For this review, take the finished solid that the model builds, in its own axes (mm). A direction names the side the tool comes from. Give positions to 0.01 mm unless a question says otherwise; leave off trailing zeros. Loops run counter-clockwise (first coordinate to the right, second up) from the corner with the lowest first, then second, coordinate; pieces in that order, holes last. Notation, with made-up numbers: (83, -0.5) -> (105, -0.5) arc R27 cw to (105, 20.5) -> close; hole circle Ø9 at (67, 40). An arc over 180 degrees is marked (long way). Write each question's results on one line, items separated by ' | '. Start each with the question number.
```python
from build123d import *

# Parameters (mm, degrees)
SKETCH1_W               = 56
SKETCH1_H               = 7.25
SKETCH1_R               = 1.6
SKETCH1_W_2             = 5
SKETCH1_H_2             = 16.75
SKETCH1_W_3             = 11.5
BOSS_EXTRUDE1_DEPTH     = 3
SKETCH2_W               = 8
SKETCH2_H               = 7
BOSS_EXTRUDE2_DEPTH     = 3
FILLET1_R               = 2
SKETCH3_W               = 16
SKETCH3_H               = 16
BOSS_EXTRUDE3_DEPTH     = 4
BOSS_EXTRUDE4_DEPTH     = 3
BOSS_EXTRUDE5_DEPTH     = 2
BOSS_EXTRUDE6_DEPTH     = 2
CHAMFER1_SIZE           = 3
SKETCH8_W               = 8
SKETCH8_H               = 10
CUT_EXTRUDE1_DEPTH      = 10
SKETCH9_R               = 1.45
BOSS_EXTRUDE7_DEPTH     = 3
SKETCH11_R              = 2.5
BOSS_EXTRUDE8_DEPTH     = 1.5
CUT_EXTRUDE3_DEPTH      = 74.518705103
CUT_EXTRUDE3_DEPTH_BACK = 2
CUT_EXTRUDE4_DEPTH      = 72.979163652
CUT_EXTRUDE4_DEPTH_BACK = 2


with BuildPart() as part:
    # Sketch1 → Boss-Extrude1 (new body)
    # profile 1 of 4: a face of its own
    with BuildSketch(Plane(origin=(0, 0, 0), x_dir=(1, 0, 0), z_dir=(0, 1, 0))):
        with Locations((-28, 3.625)):
            Rectangle(SKETCH1_W, SKETCH1_H)
        with Locations(Location((-7.6, 3.625, 0), (0, 0, 270))):
            Circle(SKETCH1_R, mode=Mode.SUBTRACT)
        with Locations(Location((-48.4, 3.625, 0), (0, 0, 270))):
            Circle(SKETCH1_R, mode=Mode.SUBTRACT)
    # profile 2 of 4: a face of its own
    with BuildSketch(Plane(origin=(0, 0, 0), x_dir=(1, 0, 0), z_dir=(0, 1, 0))):
        with Locations((-2.5, -8.375)):
            Rectangle(SKETCH1_W_2, SKETCH1_H_2)
    # profile 3 of 4: a face of its own
    with BuildSketch(Plane(origin=(0, 0, 0), x_dir=(1, 0, 0), z_dir=(0, 1, 0))):
        with Locations((5.75, -8.375)):
            Rectangle(SKETCH1_W_3, SKETCH1_H_2)
    # profile 4 of 4: a face of its own
    with BuildSketch(Plane(origin=(0, 0, 0), x_dir=(1, 0, 0), z_dir=(0, 1, 0))):
        with Locations((-10.75, -8.375)):
            Rectangle(SKETCH1_W_3, SKETCH1_H_2)
    extrude(amount=BOSS_EXTRUDE1_DEPTH)

    # Sketch2 → Boss-Extrude2 (add)
    # profile 1 of 2: a face of its own
    with BuildSketch(Plane(origin=(0, 3, 0), x_dir=(1, 0, 0), z_dir=(0, 1, 0))):
        with Locations((-48.4, 3.625)):
            Rectangle(SKETCH2_W, SKETCH2_H)
        Polygon((-46.725684219, 0.725), (-45.051368439, 3.625), (-46.725684219, 6.525), (-50.074315781, 6.525), (-51.748631561, 3.625), (-50.074315781, 0.725), align=None, mode=Mode.SUBTRACT)
    # profile 2 of 2: a face of its own
    with BuildSketch(Plane(origin=(0, 3, 0), x_dir=(1, 0, 0), z_dir=(0, 1, 0))):
        with Locations((-7.6, 3.625)):
            Rectangle(SKETCH2_W, SKETCH2_H)
        Polygon((-5.925684219, 0.725), (-4.251368439, 3.625), (-5.925684219, 6.525), (-9.274315781, 6.525), (-10.948631561, 3.625), (-9.274315781, 0.725), align=None, mode=Mode.SUBTRACT)
    extrude(amount=BOSS_EXTRUDE2_DEPTH)

    # Fillet1
    fillet1_edges = [part.edges().sort_by_distance(p)[0] for p in [
        (-44.4, 4.5, -0.125),
        (-44.4, 4.5, -7.125),
        (-52.4, 4.5, -7.125),
        (-52.4, 4.5, -0.125),
        (-3.6, 4.5, -0.125),
        (-3.6, 4.5, -7.125),
        (-11.6, 4.5, -7.125),
        (-11.6, 4.5, -0.125),
    ]]
    fillet(fillet1_edges, radius=FILLET1_R)

    # Sketch3 → Boss-Extrude3 (add)
    with BuildSketch(Plane(origin=(0, 3, 0), x_dir=(1, 0, 0), z_dir=(0, 1, 0))):
        with Locations((3.5, -8.75)):
            Rectangle(SKETCH3_W, SKETCH3_H)
    extrude(amount=BOSS_EXTRUDE3_DEPTH)

    # Sketch5 → Boss-Extrude4 (add)
    with BuildSketch(Plane.ZY.offset(4.5)):
        Polygon((-9.25, 7), (0.75, 7), (16.75, 7), (30.75, 7), (30.75, 37), (-9.25, 37), align=None)
    extrude(amount=-BOSS_EXTRUDE4_DEPTH)

    # Sketch6 → Boss-Extrude5 (add)
    with BuildSketch(Plane.XY.offset(16.75)):
        Polygon((-1.5, 37), (0, 37), (11.5, 7), (-1.5, 7), align=None)
    extrude(amount=-BOSS_EXTRUDE5_DEPTH)

    # Sketch7 → Boss-Extrude6 (add)
    with BuildSketch(Plane(origin=(0, 0, 0.75), x_dir=(-1, 0, 0), z_dir=(0, 0, -1))):
        Polygon((1.5, 37), (0, 37), (-11.5, 7), (1.5, 7), align=None)
    extrude(amount=-BOSS_EXTRUDE6_DEPTH)

    # Chamfer1
    chamfer1_edges = [part.edges().sort_by_distance(p)[0] for p in [
        (-3, 7, -9.25),
        (-3, 37, -9.25),
        (-3, 37, 30.75),
        (-3, 7, 30.75),
    ]]
    chamfer(chamfer1_edges, length=CHAMFER1_SIZE)

    # Sketch8 → Cut-Extrude1 (cut)
    with BuildSketch(Plane(origin=(-1.5, 0, 0), x_dir=(0, 0, -1), z_dir=(1, 0, 0))):
        with Locations((-8.75, 22)):
            Rectangle(SKETCH8_W, SKETCH8_H)
    extrude(amount=-CUT_EXTRUDE1_DEPTH, mode=Mode.SUBTRACT)

    # Sketch9 → Boss-Extrude7 (add)
    with BuildSketch(Plane(origin=(-1.5, 0, 0), x_dir=(0, 0, -1), z_dir=(1, 0, 0))):
        with Locations(Location((-8.75, 31.75, 0), (0, 0, 180))):
            Circle(SKETCH9_R)
        with Locations(Location((-8.75, 12.25, 0), (0, 0, 180))):
            Circle(SKETCH9_R)
    extrude(amount=BOSS_EXTRUDE7_DEPTH)

    # Sketch11 → Boss-Extrude8 (add)
    with BuildSketch(Plane(origin=(-1.5, 0, 0), x_dir=(0, 0, -1), z_dir=(1, 0, 0))):
        with Locations(Location((-8.75, 31.75, 0), (0, 0, 180))):
            Circle(SKETCH11_R)
        with Locations(Location((-8.75, 12.25, 0), (0, 0, 180))):
            Circle(SKETCH11_R)
    extrude(amount=BOSS_EXTRUDE8_DEPTH)

    # Sketch13 → Cut-Extrude3 (cut, two sides: drawn at the far end of the back side and taken through both)
    with BuildSketch(Plane(origin=(0, 0, 0.75), x_dir=(-1, 0, 0), z_dir=(0, 0, -1)).offset(-CUT_EXTRUDE3_DEPTH_BACK)):
        Polygon((0, 185.220530074), (0, 37), (0, 13.52173913), (-9, 13.52173913), (-157.220530074, 13.52173913), (-375.851096448, 213.716588185), (-218.630566375, 385.415379128), align=None)
    extrude(amount=CUT_EXTRUDE3_DEPTH + CUT_EXTRUDE3_DEPTH_BACK, mode=Mode.SUBTRACT)

    # Sketch14 → Cut-Extrude4 (cut, two sides: drawn at the far end of the back side and taken through both)
    with BuildSketch(Plane.XY.offset(16.75).offset(-CUT_EXTRUDE4_DEPTH_BACK)):
        Polygon((0, 185.220530074), (0, 37), (0, 13.52173913), (9, 13.52173913), (157.220530074, 13.52173913), (375.851096448, 213.716588185), (218.630566375, 385.415379128), align=None)
    extrude(amount=CUT_EXTRUDE4_DEPTH + CUT_EXTRUDE4_DEPTH_BACK, mode=Mode.SUBTRACT)


solid = part.part
```
1. We need section C-C (x = -7.6). Write out the cut boundary in (y, z) (3 decimals).
2. For pin 1 Ø8 at (y, z) = (25.5, 20) entering from -X; pin 2 Ø4 at (x, y) = (3.5, 24) entering from -Z; pin 3 Ø8 at (x, y) = (4, 12) entering from -Z; pin 4 Ø1.5 at (x, y) = (-8, 5) entering from -Z (3 decimals), all flat-tipped, find the tip position at first contact; note any pin that passes through.
3. We need section B-B (y = 23). Write out the cut boundary in (x, z).
4. We need section D-D (z = 13.5). Write out the cut boundary in (x, y), plus the area to 3 significant figures.
5. Machinability: for faces 4 (the cylindrical face through (-10.999, 4.521, -6.555)), 5 (the cylindrical face through (-45.001, 4.521, -0.695)), 6 (the flat face through (-45.9, 4.479, -2.155)), 7 (the flat face through (-3.6, 4, -4)), 8 (the flat face through (0, 25, 2)), which of the approach directions +Z, -Z, +X, -X, +Y, -Y give a long, thin tool a straight path to every point of the face, cutting with its end or side? Answer none if there is none.
6. Wall thickness on L1, parallel to Y at x = -2.5, z = -4; L2, parallel to Z at x = -3.5, y = 20; L3, parallel to X at y = 30, z = 19: over which ranges is each line inside the solid? List them lowest first.
7. Draft analysis for pull direction Y (two halves, no side actions). For faces 1 (the cylindrical face through (-46.814, 1.479, -3.833)), 2 (the flat face through (-10.3, 6, -2.1)), 3 (the flat face through (5, 13.522, 2)), state which applies: released by +Y, released by -Y, zero draft, split by the parting line, or undercut.
8. We need section A-A (z = 8.75). Write out the cut boundary in (x, y).
Response:
1) outline: (0, -7.25) -> (3, -7.25) -> (3, -7.125) -> (6, -7.125) -> (6, -6.525) -> (3, -6.525) -> (3, -5.225) -> (0, -5.225) -> close; (0, -2.025) -> (3, -2.025) -> (3, -0.725) -> (6, -0.725) -> (6, -0.125) -> (3, -0.125) -> (3, 16.75) -> (0, 16.75) -> close
2) pin 1: stops at x = -4.5 | pin 2: passes through | pin 3: stops at z = 0.75 | pin 4: stops at z = -7.125
3) outline: (-4.5, -9.25) -> (-1.5, -9.25) -> (-1.5, 0.75) -> (0, 0.75) -> (0, 2.75) -> (-1.5, 2.75) -> (-1.5, 4.75) -> (-4.5, 4.75) -> close; (-4.5, 12.75) -> (-1.5, 12.75) -> (-1.5, 14.75) -> (0, 14.75) -> (0, 16.75) -> (-1.5, 16.75) -> (-1.5, 30.75) -> (-4.5, 30.75) -> close
4) outline: (-16.5, 0) -> (11.5, 0) -> (11.5, 7) -> (-1.5, 7) -> (-1.5, 37) -> (-4.5, 37) -> (-4.5, 3) -> (-16.5, 3) -> close | area: 238 mm2
5) face 4: -Z, +Y | face 5: +Z, +Y | face 6: +Y | face 7: -Z, +X | face 8: -Z, +X, +Y
6) L1: y = 0 to 3, 7 to 37 | L2: z = -9.25 to 4.75, 12.75 to 30.75 | L3: x = -4.5 to -1.5
7) face 1: zero draft | face 2: undercut | face 3: released by +Y
8) outline: (-16.5, 0) -> (11.5, 0) -> (11.5, 7) -> (-1.5, 7) -> (-1.5, 9.75) -> (0, 9.75) -> (0, 10.8) -> (1.5, 10.8) -> (1.5, 13.7) -> (0, 13.7) -> (0, 14.75) -> (-1.5, 14.75) -> (-1.5, 17) -> (-4.5, 17) -> (-4.5, 3) -> (-16.5, 3) -> close; (-4.5, 27) -> (-1.5, 27) -> (-1.5, 29.25) -> (0, 29.25) -> (0, 30.3) -> (1.5, 30.3) -> (1.5, 33.2) -> (0, 33.2) -> (0, 34.25) -> (-1.5, 34.25) -> (-1.5, 37) -> (-4.5, 37) -> close
